from build123d import *

# Parameters (mm, degrees)
F1_DEPTH = 31.75
F2_W     = 24.130002
F2_H     = 12.7
F3_DEPTH = 12.7
F4_R     = 7.874
F5_DEPTH = 12.7


with BuildPart() as f1:
    # F0 (on Front) → F1 (new body)
    with BuildSketch(Plane.XZ):
        Polygon((0, 12.7), (0, 0), (47.752, 0), (54.102, 19.05), (88.9, 19.05), (88.9, 31.75), (44.45, 31.75), (38.1, 12.7), align=None)
    extrude(amount=F1_DEPTH)

    # F2 (on face) → F3 (cut)
    with BuildSketch(Plane.XY.offset(31.75)):
        with Locations((76.834999, -15.875)):
            Rectangle(F2_W, F2_H)
    extrude(amount=-F3_DEPTH, mode=Mode.SUBTRACT)

    # F4 (on face) → F5 (cut)
    with BuildSketch(Plane.XY.offset(12.7)):
        with Locations((19.05, -15.748)):
            Circle(F4_R)
    extrude(amount=-F5_DEPTH, mode=Mode.SUBTRACT)


solid = f1.part
Geometry: final body of the model. Coordinates: model frame, mm. A direction names the side the tool comes from. Coordinates: 2 decimals unless noted, no trailing zeros. Loops run counter-clockwise (first coordinate to the right, second up) from the corner with the lowest first, then second, coordinate; pieces in that order, holes last. Notation, with made-up numbers: (-25.75, 79.25) - (33.25, 79.25) arc R28 cw to (33.25, 105.25) - close; hole circle Ø5 at (83.25, 70). An arc over 180 degrees is marked (long way). One line per question, with ' | ' between items. Start each with the question number.
(1) Cut plane C-C on x = 19.05. Output: boundary loops of the cut face in (y, z), and give its area (3 significant figures).
(2) Cut plane B-B on y = -20. Output: boundary loops of the cut face in (x, z), and give its area (3 significant figures).
(3) Cut plane A-A on x = 71.5. Output: boundary loops of the cut face in (y, z) (3 decimals), and give its area (3 significant figures).
(4) Draft query along Y for faces 1 (the flat face through (44, 0, 16)), 2 (the flat face through (29, -16, 0)), 3 (the flat face through (77, -22.225, 25)), 4 (the flat face through (44, -31.75, 16)). Return one class per face: +Y half, -Y half, draft (parallel to the pull), parting line (faces both ways), or undercut.
(5) Ray query, L1, parallel to Y at x = 82, z = 24.5 (3 decimals); L2, parallel to Z at x = 29.5, y = -2; L3, parallel to Z at x = 74, y = -6. Return the intervals inside material, ascending. Write a range as from..to.
(6) Cut plane D-D on z = 3. Output: boundary loops of the cut face in (x, y).
(7) Reachability of faces 5 (the flat face through (88.9, -5, 25)), 6 (the flat face through (77, -9.525, 25)), 7 (the flat face through (64, -16, 19.05)), 8 (the flat face through (24, -23, 12.7)) from +Z, -Z, +X, -X, +Y, -Y: full face, straight path, thin tool, end or side. Return the list, or none.
(8) First-contact query: pin 1 (16 mm diameter, centred on x = 75.5, y = -10.5, fed in from -Z); pin 2 (1 mm diameter, centred on y = -26, z = 16, fed in from +X); pin 3 (12 mm diameter, centred on x = 23.5, y = -20.5, fed in from +Z). Flat tips, straight axial feed; report the tip coordinate or a pass-through.
Here are the results:
1) outline: (-31.75, 0) - (-23.62, 0) - (-23.62, 12.7) - (-31.75, 12.7) - close; (-7.87, 0) - (0, 0) - (0, 12.7) - (-7.87, 12.7) - close | area: 203 mm²
2) outline: (0, 0) - (12.42, 0) - (12.42, 12.7) - (0, 12.7) - close; (25.68, 0) - (47.75, 0) - (54.1, 19.05) - (64.77, 19.05) - (64.77, 31.75) - (44.45, 31.75) - (38.1, 12.7) - (25.68, 12.7) - close | area: 838 mm²
3) outline: (-31.75, 19.05) - (-22.225, 19.05) - (-22.225, 31.75) - (-31.75, 31.75) - close; (-9.525, 19.05) - (0, 19.05) - (0, 31.75) - (-9.525, 31.75) - close | area: 242 mm²
4) face 1: +Y half | face 2: draft | face 3: undercut | face 4: -Y half
5) L1: -31.75..-22.225, -9.525..0 | L2: 0..12.7 | L3: 19.05..31.75
6) outline: (0, -31.75) - (48.75, -31.75) - (48.75, 0) - (0, 0) - close; hole circle Ø15.75 at (19.05, -15.75)
7) face 5: +Z, -Z, +X, +Y, -Y | face 6: +Z, -Z, +X | face 7: -Z, +X, +Y, -Y | face 8: +Z, -X, +Y, -Y
8) pin 1: z = 19.05 | pin 2: x = 53.25 | pin 3: z = 12.7
